Check sheet for the modelled part. Datum: model origin and axes. Units: mm. A direction names the side the tool comes from. Coordinates: 2 decimals unless noted, no trailing zeros. Loops run counter-clockwise (first coordinate to the right, second up) from the corner with the lowest first, then second, coordinate; pieces in that order, holes last. Notation, with made-up numbers: M -7.5,15 L 38.5,15 A10 cw 38.5,19 Z; hole C 17.25,41.25 d4. An arc over 180 degrees is marked long. Return JSON: item names as keys, results as strings.
from build123d import *

# Parameters (mm, degrees)
F0_R     = 13
F1_DEPTH = 2.5
F2_R     = 5
F3_DEPTH = 3.5
F4_R     = 4.745
F5_DEPTH = 7
F6_R     = 1


with BuildPart() as f1:
    # F0 (on Top) → F1 (new body)
    with BuildSketch(Plane.XY):
        Circle(F0_R)
    extrude(amount=F1_DEPTH)

    # F2 (on Top) → F3 (join)
    with BuildSketch(Plane.XY):
        Circle(F2_R)
    extrude(amount=F3_DEPTH)

    # F4 (on Top) → F5 (join)
    with BuildSketch(Plane.XY):
        Circle(F4_R)
    extrude(amount=F5_DEPTH)

    # F6
    f6_edges = [f1.edges().sort_by_distance(p)[0] for p in [
        (-4.745, 0, 7),
    ]]
    fillet(f6_edges, radius=F6_R)


solid = f1.part
1) Set-up check for faces 1 (the face through (0, 0, 0)), 2 (the face through (6, 0, 2.5)): record each of +Z, -Z, +X, -X, +Y, -Y from which the full face is reachable in a straight line by a thin tool's end or side.
Answers:
{"face 1": "-Z, +X, -X, +Y, -Y", "face 2": "+Z"}
2) Scan lines: line 1 along Z through (x, y) = (-0.5, -10.5); line 2 along Y through (x, z) = (11, 1.5); line 3 along Z through (x, y) = (-3.5, 1.75). Record each from-to range of solid material in increasing order. Write a range as [from, to].
Answers:
{"line 1": "[0, 2.5]", "line 2": "[-6.93, 6.93]", "line 3": "[0, 6.99]"}
3) Section check D-D on z = 1.25. Record the cut outline in (x, y).
Answers:
{"outline": "C 0,0 d26"}
4) Section check C-C on z = 4.5. Record the cut outline in (x, y) (3 decimals), then the cut area to 3 significant figures.
Answers:
{"outline": "C 0,0 d9.49", "area": "70.7 mm²"}
5) Section check A-A on x = 0. Record the cut outline in (y, z) (3 decimals), then the cut area to 3 significant figures.
Answers:
{"outline": "M -13,0 L 13,0 L 13,2.5 L 5,2.5 L 5,3.5 L 4.745,3.5 L 4.745,6 A1 ccw 3.745,7 L -3.745,7 A1 ccw -4.745,6 L -4.745,3.5 L -5,3.5 L -5,2.5 L -13,2.5 Z", "area": "108 mm²"}
